CAD build for the part. Positions are in the model's coordinates, mm. Round coordinates to 2 decimals unless told otherwise and drop trailing zeros. Order: outer loops, then holes, each group sorted by start corner. A loop starts at its lowest first (then second) coordinate and runs counter-clockwise, first axis right, second up. Notation, with made-up numbers: (-39.75, 73) -> (-19.75, 73) arc R18 cw to (-19.75, 107) -> close; hole circle Ø4 at (-23, 2). An arc over 180 degrees is marked (long way). Answer as CSV lines item,"result". Start each with the question number.
from build123d import *

# Parameters (mm, degrees)
F0_R     = 0.9217746556
F0_W     = 51.8037118018
F0_H     = 75.0324204564
F0_R_2   = 3.4304363285
F1_DEPTH = 1.27
F2_DEPTH = 7.62


with BuildPart() as f1:
    # F0 (on Front) → F1 (new body)
    with BuildSketch(Plane.XZ):
        with BuildLine():
            ThreePointArc((-28.3087114036, 46.0887122899), (-32.7988394641, 44.2288403505), (-34.6587114036, 39.7387122899))
            Line((-34.6587114036, 39.7387122899), (-34.6587114036, 36.3179035485))
            Line((-34.6587114036, 36.3179035485), (17.1450003982, 36.3179035485))
            Line((17.1450003982, 36.3179035485), (17.1450003982, 39.7387122899))
            ThreePointArc((17.1450003982, 39.7387122899), (15.2851284587, 44.2288403505), (10.7950003982, 46.0887122899))
            Line((10.7950003982, 46.0887122899), (-28.3087114036, 46.0887122899))
        make_face()
        with Locations((-20.6477418542, 42.032904923)):
            Circle(F0_R, mode=Mode.SUBTRACT)
        with Locations((-8.7568555027, -1.1983066797)):
            Rectangle(F0_W, F0_H)
        with BuildLine():
            Line((17.1450003982, -38.7145169079), (-34.6587114036, -38.7145169079))
            Line((-34.6587114036, -38.7145169079), (-34.6587114036, -44.7162905872))
            ThreePointArc((-34.6587114036, -44.7162905872), (-32.7988394641, -49.2064186477), (-28.3087114036, -51.0662905872))
            Line((-28.3087114036, -51.0662905872), (10.7950003982, -51.0662905872))
            ThreePointArc((10.7950003982, -51.0662905872), (15.2851284587, -49.2064186477), (17.1450003982, -44.7162905872))
            Line((17.1450003982, -44.7162905872), (17.1450003982, -38.7145169079))
        make_face()
        with Locations((-8.7568555027, -43.6921007931)):
            Circle(F0_R_2, mode=Mode.SUBTRACT)
    extrude(amount=F1_DEPTH)

    # F0 (on Front) → F2 (join)
    with BuildSketch(Plane.XZ):
        with BuildLine():
            ThreePointArc((-28.3087114036, 46.0887122899), (-32.7988394641, 44.2288403505), (-34.6587114036, 39.7387122899))
            Line((-34.6587114036, 39.7387122899), (-34.6587114036, 36.3179035485))
            Line((-34.6587114036, 36.3179035485), (17.1450003982, 36.3179035485))
            Line((17.1450003982, 36.3179035485), (17.1450003982, 39.7387122899))
            ThreePointArc((17.1450003982, 39.7387122899), (15.2851284587, 44.2288403505), (10.7950003982, 46.0887122899))
            Line((10.7950003982, 46.0887122899), (-28.3087114036, 46.0887122899))
        make_face()
        with Locations((-20.6477418542, 42.032904923)):
            Circle(F0_R, mode=Mode.SUBTRACT)
        with Locations((-8.7568555027, -1.1983066797)):
            Rectangle(F0_W, F0_H)
        with BuildLine():
            Line((17.1450003982, -38.7145169079), (-34.6587114036, -38.7145169079))
            Line((-34.6587114036, -38.7145169079), (-34.6587114036, -44.7162905872))
            ThreePointArc((-34.6587114036, -44.7162905872), (-32.7988394641, -49.2064186477), (-28.3087114036, -51.0662905872))
            Line((-28.3087114036, -51.0662905872), (10.7950003982, -51.0662905872))
            ThreePointArc((10.7950003982, -51.0662905872), (15.2851284587, -49.2064186477), (17.1450003982, -44.7162905872))
            Line((17.1450003982, -44.7162905872), (17.1450003982, -38.7145169079))
        make_face()
        with Locations((-8.7568555027, -43.6921007931)):
            Circle(F0_R_2, mode=Mode.SUBTRACT)
    extrude(amount=F2_DEPTH)


solid = f1.part
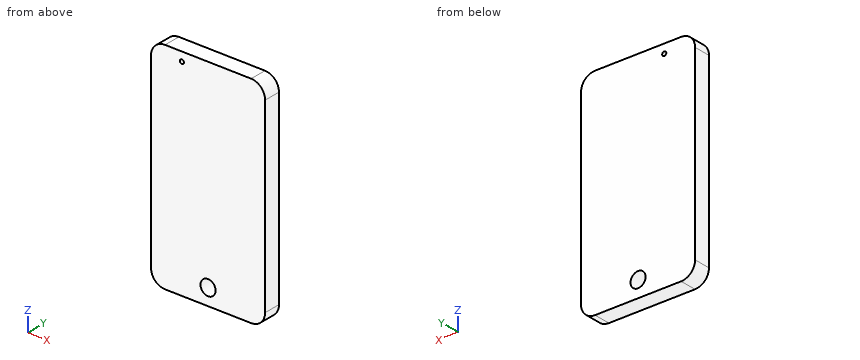
Item 1: Band-saw the part on A-A, the plane x = -10. Give the cut face in (y, z), and give its area (3 significant figures).
Item 2: Pin check, flat tip, straight feed: pin 1 (4 mm diameter, centred on x = -8.76, z = -43.69, fed in from -Y). Stop position of the tip, or through.
Item 3: Band-saw the part on B-B, the plane z = -42. Give the cut face in (x, y) (3 decimals).
Item 4: Probe line 1 (Z direction, x = -20.5, y = -2); line 2 (Z direction, x = -11, y = -4.25); line 3 (X direction, y = -5.5, z = 40). List the from-to ranges inside material, lowest first.
Values:
1,outline,"(-7.62, -51.07) -> (0, -51.07) -> (0, -46.89) -> (-7.62, -46.89) -> close; (-7.62, -40.49) -> (0, -40.49) -> (0, 46.09) -> (-7.62, 46.09) -> close"
1,area,"692 mm²"
2,pin 1,"through"
3,outline,"(-34.659, -7.62) -> (-11.741, -7.62) -> (-11.741, 0) -> (-34.659, 0) -> close; (-5.773, -7.62) -> (17.145, -7.62) -> (17.145, 0) -> (-5.773, 0) -> close"
4,line 1,"-51.07 to 41.12, 42.94 to 46.09"
4,line 2,"-51.07 to -46.29, -41.1 to 46.09"
4,line 3,"-34.65 to 17.14"
